Autodesk Inventor part; units mm, degrees
ref_plane "YZ Plane" through (0, 0, 0) normal (1, 0, 0) x (0, 1, 0)
ref_plane "XZ Plane" through (0, 0, 0) normal (0, 1, 0) x (-1, 0, 0)
ref_plane "XY Plane" through (0, 0, 0) normal (0, 0, 1) x (1, 0, 0)
sketch "Sketch1" plane through (0, 0, 0) normal (0, 0, 1) x (1, 0, 0)
  line L0 (3.175, 0) -> (22.225, 0)
  line L1 (25.4, 3.175) -> (25.4, 47.625)
  line L2 (22.225, 50.8) -> (3.175, 50.8)
  line L3 (0, 47.625) -> (0, 3.175)
  arc A0 (3.175, 50.8) -> (0, 47.625) centre (3.175, 47.625) ccw
  arc A1 (25.4, 47.625) -> (22.225, 50.8) centre (22.225, 47.625) ccw
  arc A2 (22.225, 0) -> (25.4, 3.175) centre (22.225, 3.175) ccw
  arc A3 (0, 3.175) -> (3.175, 0) centre (3.175, 3.175) ccw
  line L4 (6.35, 47.625) -> (19.05, 47.625)
  line L5 (22.225, 44.45) -> (22.225, 6.35)
  line L6 (19.05, 3.175) -> (6.35, 3.175)
  line L7 (3.175, 6.35) -> (3.175, 44.45)
  arc A4 (6.35, 47.625) -> (3.175, 44.45) centre (6.35, 44.45) ccw
  arc A5 (22.225, 44.45) -> (19.05, 47.625) centre (19.05, 44.45) ccw
  arc A6 (3.175, 6.35) -> (6.35, 3.175) centre (6.35, 6.35) ccw
  arc A7 (19.05, 3.175) -> (22.225, 6.35) centre (19.05, 6.35) ccw
  point P0 (0, 0)
  point P1 (25.4, 0)
  point P2 (0, 50.8)
  dimension "d0" = 50.8
  dimension "d1" = 25.4
  dimension "d2" = 3.175
  dimension "d3" = 3.175
  dimension "d4" = 3.175
  dimension "d5" = 3.175
  dimension "d6" = 3.175
  dimension "d7" = 3.175
  dimension "d8" = 3.175
  dimension "d9" = 3.175
  dimension "d10" = 3.175
extrude "Extrusion1" add sketch "Sketch1" along normal blind 101.6
properties part number "O channel 4 inch"
The listing builds one solid part. Answer for the finished solid, in the listing's coordinates (mm). A direction names the side the tool comes from. Give positions to 0.01 mm unless a question says otherwise; leave off trailing zeros. Order: outer loops, then holes, each group sorted by start corner. A loop starts at its lowest first (then second) coordinate and runs counter-clockwise, first axis right, second up. Notation, with made-up numbers: (58.25, 16) -> (109.25, 16) arc R23 cw to (109.25, 50) -> close; hole circle Ø7 at (33.25, 26.25). An arc over 180 degrees is marked (long way). Answer as CSV lines item,"result". Start each with the question number.
Q1. A cutting plane is placed at B-B (y = 12). Determine the outline of the cut face in (x, z) (3 decimals), then the cut area to 3 significant figures.
Q2. Determine the mould class of faces 1 (the cylindrical face through (0.91, 49.85, 50.09)), 2 (the cylindrical face through (4.13, 4.08, 50.09)), 3 (the flat face through (13, 47.625, 50)), 4 (the cylindrical face through (0.95, 0.91, 50.09)) for opening direction Y: pulls with the +Y half, pulls with the -Y half, needs draft (parallel to the pull), parting line crosses it, or undercut.
Q3. A cutting plane is placed at A-A (x = 13.5). Determine the outline of the cut face in (y, z) (3 decimals), then the cut area to 3 significant figures.
Q4. A cutting plane is placed at C-C (z = 19.5). Determine the outline of the cut face in (x, y) (3 decimals).
Q5. Find the intervals of material crossed by L1, parallel to X at y = 22.5, z = 34 (3 decimals); L2, parallel to Y at x = 7.5, z = 76 (3 decimals); L3, parallel to X at y = 3, z = 81, in increasing order.
Q6. Which of the six approach directions +Z, -Z, +X, -X, +Y, -Y give full straight-line access (tool end or side, diameter ignored) to faces 5 (the cylindrical face through (4.08, 46.67, 50.09)), 6 (the cylindrical face through (24.45, 49.89, 50.09))?
Results found:
1,outline,"(0, 0) -> (3.175, 0) -> (3.175, 101.6) -> (0, 101.6) -> close; (22.225, 0) -> (25.4, 0) -> (25.4, 101.6) -> (22.225, 101.6) -> close"
1,area,"645 mm2"
2,face 1,"pulls with the +Y half"
2,face 2,"undercut"
2,face 3,"undercut"
2,face 4,"pulls with the -Y half"
3,outline,"(0, 0) -> (3.175, 0) -> (3.175, 101.6) -> (0, 101.6) -> close; (47.625, 0) -> (50.8, 0) -> (50.8, 101.6) -> (47.625, 101.6) -> close"
3,area,"645 mm2"
4,outline,"(0, 3.175) arc R3.175 ccw to (3.175, 0) -> (22.225, 0) arc R3.175 ccw to (25.4, 3.175) -> (25.4, 47.625) arc R3.175 ccw to (22.225, 50.8) -> (3.175, 50.8) arc R3.175 ccw to (0, 47.625) -> close; hole (3.175, 6.35) arc R3.175 ccw to (6.35, 3.175) -> (19.05, 3.175) arc R3.175 ccw to (22.225, 6.35) -> (22.225, 44.45) arc R3.175 ccw to (19.05, 47.625) -> (6.35, 47.625) arc R3.175 ccw to (3.175, 44.45) -> close"
5,L1,"0 to 3.175, 22.225 to 25.4"
5,L2,"0 to 3.175, 47.625 to 50.8"
5,L3,"0 to 25.4"
6,face 5,"+Z, -Z"
6,face 6,"+Z, -Z, +X, +Y"
